Input: part model. Units: mm. Frame: model coordinates. Give positions to 0.01 mm unless a question says otherwise; leave off trailing zeros. Loops run counter-clockwise (first coordinate to the right, second up) from the corner with the lowest first, then second, coordinate; pieces in that order, holes last. Notation, with made-up numbers: (-13.5, 24) -> (29.5, 24) arc R19 cw to (29.5, 33) -> close; hole circle Ø4 at (25.5, 54.5). An arc over 180 degrees is marked (long way). One line per question, with ' | ' between items.
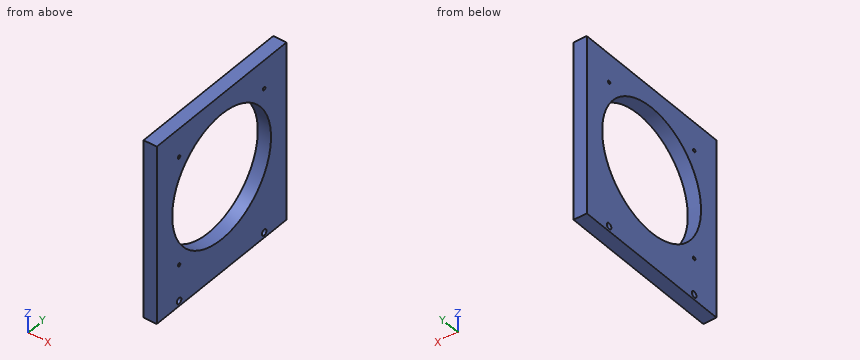
from build123d import *

# Parameters (mm, degrees)
SKETCH1_W           = 86.36
SKETCH1_H           = 80
SKETCH1_R           = 30.5
BOSS_EXTRUDE1_DEPTH = 6.35
SKETCH3_R           = 0.762
SKETCH3_R_2         = 1.4224
CUT_EXTRUDE2_DEPTH  = 6.35


with BuildPart() as part:
    # Sketch1 → Boss-Extrude1 (new body)
    with BuildSketch(Plane(origin=(0, 0, 0), x_dir=(0, 0, -1), z_dir=(1, 0, 0))):
        with Locations((43.18, 40)):
            Rectangle(SKETCH1_W, SKETCH1_H)
        with Locations((40, 40)):
            Circle(SKETCH1_R, mode=Mode.SUBTRACT)
    extrude(amount=BOSS_EXTRUDE1_DEPTH)

    # Sketch3 → Cut-Extrude2 (cut)
    with BuildSketch(Plane.ZY):
        with Locations((-66.292558248, 13.75)):
            Circle(SKETCH3_R)
        with Locations((-13.754723938, 13.75)):
            Circle(SKETCH3_R)
        with Locations((-13.754723938, 66.25)):
            Circle(SKETCH3_R)
        with Locations((-83.82, 13.75)):
            Circle(SKETCH3_R_2)
        with Locations((-83.82, 66.25)):
            Circle(SKETCH3_R_2)
    extrude(amount=-CUT_EXTRUDE2_DEPTH, mode=Mode.SUBTRACT)


solid = part.part
1. Ray query, line 1 along Y through (x, z) = (4, -83.82); line 2 along Z through (x, y) = (3.5, 39.5); line 3 along Y through (x, z) = (0.75, -45). Return the intervals inside material, ascending. Write a range as from..to.
Determined:
line 1: y = 0..12.33, 15.17..64.83, 67.67..80 | line 2: z = -86.36..-70.5, -9.5..0 | line 3: y = 0..9.91, 70.09..80
2. Section query A-A (z = -83.82). Output: boundary loops of the cut face in (x, y), then the cut area to 3 significant figures.
Determined:
outline: (0, 0) -> (6.35, 0) -> (6.35, 12.33) -> (0, 12.33) -> close; (0, 15.17) -> (6.35, 15.17) -> (6.35, 64.83) -> (0, 64.83) -> close; (0, 67.67) -> (6.35, 67.67) -> (6.35, 80) -> (0, 80) -> close | area: 472 mm2
3. Section query B-B (z = -40). Output: boundary loops of the cut face in (x, y).
Determined:
outline: (0, 0) -> (6.35, 0) -> (6.35, 9.5) -> (0, 9.5) -> close; (0, 70.5) -> (6.35, 70.5) -> (6.35, 80) -> (0, 80) -> close
4. Section query D-D (y = 40). Output: boundary loops of the cut face in (x, z).
Determined:
outline: (0, -86.36) -> (6.35, -86.36) -> (6.35, -70.5) -> (0, -70.5) -> close; (0, -9.5) -> (6.35, -9.5) -> (6.35, 0) -> (0, 0) -> close
5. Section query C-C (x = 3.75). Output: boundary loops of the cut face in (y, z), then the cut area to 3 significant figures.
Determined:
outline: (0, -86.36) -> (80, -86.36) -> (80, 0) -> (0, 0) -> close; hole circle Ø61 at (40, -40); hole circle Ø2.84 at (13.75, -83.82); hole circle Ø1.52 at (13.75, -66.29); hole circle Ø1.52 at (13.75, -13.75); hole circle Ø2.84 at (66.25, -83.82); hole circle Ø1.52 at (66.25, -13.75) | area: 3,970 mm2
